Verification items for the finished model (mm, model axes). A direction names the side the tool comes from. Coordinates: 2 decimals unless noted, no trailing zeros. Loops run counter-clockwise (first coordinate to the right, second up) from the corner with the lowest first, then second, coordinate; pieces in that order, holes last.
Q1. Go/stop test with flat-tipped pins: P1, Ø8.5, axis at x = 5.5, y = 49, coming from the +Z side; P2, Ø4, axis at x = -18.85, y = -42.07, coming from the +Z side. Record where each tip stops, or that it passes through.
Q2. Material ranges on probe 1 along X at (y, z) = (94, 6.25); probe 2 along X at (y, z) = (140.5, 10.5); probe 3 along Y at (x, z) = (18, 12), recorded low to high.
Q3. Sectioned sample at A-A (z = 12.5). Count the separate pieces of the cut face and the enclosed holes in it, then the cut area to 3 significant figures.
Q4. Access from +Z, -Z, +X, -X, +Y, -Y to the whole of each face (thin tool, end or side, straight path). Record for faces 4 (the face through (17, 43, 7.938)), 5 (the face through (40.96, 65.94, 8.05)).
Q5. Mould release check, pull along Y, two halves, no side actions. Record for faces 1 (the face through (11, -52.388, 8)), 2 (the face through (10.282, 57.082, 4.024)), 3 (the face through (11, 143, 15.875)): +Y half, -Y half, draft (parallel to the pull), parting line (faces both ways), or undercut.
Q6. Sectioned sample at C-C (y = 54). Enter the section's corners in (x, z) (1 decimal), then the cut area to 3 significant figures.
Autodesk Inventor part; units mm, degrees
ref_plane "YZ Plane" through (0, 0, 0) normal (1, 0, 0) x (0, 1, 0)
ref_plane "XZ Plane" through (0, 0, 0) normal (0, 1, 0) x (-1, 0, 0)
ref_plane "XY Plane" through (0, 0, 0) normal (0, 0, 1) x (1, 0, 0)
sketch "Sketch1" plane through (0, 0, 0) normal (0, 0, 1) x (1, 0, 0)
  line L0 (-23.6094, 98.425) -> (-0.1834, 98.425)
  line L1 (-0.1834, 150.8125) -> (-0.1834, 98.425)
  line L2 (-23.6094, 150.8125) -> (-0.1834, 150.8125)
  line L3 (-23.6094, 150.8125) -> (-23.6094, 98.425)
  circle A0 centre (-18.8469, 140.4937) radius 2.3813
  circle A1 centre (-18.8469, 108.7437) radius 2.3812
  line L4 (-23.6094, -52.3875) -> (-0.1834, -52.3875)
  line L5 (-0.1834, 0) -> (-0.1834, -52.3875)
  line L6 (-23.6094, 0) -> (0, 0)
  line L7 (-23.6094, 0) -> (-23.6094, -52.3875)
  circle A2 centre (-18.8469, -10.3188) radius 2.3813
  circle A3 centre (-18.8469, -42.0688) radius 2.3813
  line L8 (22.8147, 98.425) -> (46.2406, 98.425)
  line L9 (46.2406, 150.8125) -> (46.2406, 98.425)
  line L10 (22.8147, 150.8125) -> (46.2406, 150.8125)
  line L11 (22.8147, 150.8125) -> (22.8147, 98.425)
  circle A4 centre (41.4781, 140.4938) radius 2.3813
  circle A5 centre (41.4781, 108.7438) radius 2.3813
  line L12 (22.8147, -52.3875) -> (46.2406, -52.3875)
  line L13 (46.2406, 0) -> (46.2406, -52.3875)
  line L14 (22.8147, 0) -> (46.2406, 0)
  line L15 (22.8147, 0) -> (22.8147, -52.3875)
  circle A6 centre (41.4781, -10.3187) radius 2.3813
  circle A7 centre (41.4781, -42.0687) radius 2.3813
  line L16 (22.8147, 150.8125) -> (-0.1834, 150.8125)
  line L17 (22.8147, -52.3875) -> (-0.1834, -52.3875)
  line L18 (46.2406, 0) -> (46.2406, 98.425)
  line L19 (-23.6094, 0) -> (-23.6094, 98.425)
extrude "Extrusion1" add sketch "Sketch1" along normal blind 15.875
sketch "Sketch2" plane through (-23.6094, -52.3875, 0) normal (-1, 0, 0) x (0, 0, 1)
  line L0 (15.875, 195.2625) -> (15.875, 190.5)
  line L1 (15.875, 163.5125) -> (15.875, 158.75)
  line L2 (15.875, 44.45) -> (15.875, 39.6875)
  line L3 (15.875, 190.5) -> (15.875, 163.5125) construction
  line L4 (15.875, 12.7) -> (0, 12.7) construction
  line L5 (15.875, 12.7) -> (15.875, 39.6875) construction
  line L6 (22.1465, 177.0062) -> (15.875, 177.0062)
  line L7 (15.875, 0) -> (15.875, 203.2)
  line L8 (24.8676, 26.1938) -> (15.875, 26.1938)
  line L9 (15.875, 203.2) -> (15.875, 0)
  circle A0 centre (15.875, 177.0062) radius 9.525
  circle A1 centre (15.875, 26.1938) radius 9.525
  point P0 (0, 52.3875)
  point P1 (15.875, 35.7188)
  point P2 (15.875, 16.6688)
  point P3 (15.875, 186.5312)
  point P4 (15.875, 167.4812)
  dimension "d2" = 19.05
  dimension "d3" = 19.05
extrude "Extrusion2" cut sketch "Sketch2" against normal blind 76.2 contours L7 A1 | A0 L7 picked at (15.1152, 19.9361) picked at (15.1152, 170.7485)
sketch "Sketch3" plane through (0, 0, 15.875) normal (0, 0, 1) x (1, 0, 0)
  circle A0 centre (41.4781, 108.7438) radius 2.3813 construction
  circle A1 centre (41.4781, -10.3187) radius 2.3813 construction
  line L0 (41.4781, 108.7438) -> (41.4781, -10.3187) construction
  circle A2 centre (41.4781, 49.2125) radius 2.3813 construction
  circle A3 centre (41.4781, 30.1625) radius 2.3813 construction
  circle A4 centre (41.4781, 68.2625) radius 2.3813 construction
  circle A5 centre (41.4781, 49.2125) radius 2.3813 construction
  circle A6 centre (41.4781, 68.2625) radius 2.3813
  circle A7 centre (41.4781, 49.2125) radius 2.3813
  circle A8 centre (41.4781, 30.1625) radius 2.3813
  point P0 (0, 0)
  dimension "d8" = 19.05
  dimension "d11" = 19.05
extrude "Extrusion3" cut sketch "Sketch3" against normal blind 76.2
sketch "Sketch4" plane through (0, 0, 15.875) normal (0, 0, 1) x (1, 0, 0)
  circle A0 centre (11.3156, 49.2125) radius 14.2875
  line L0 (-23.6094, 115.0937) -> (-23.6094, -16.6688)
  point P0 (0, 0)
  dimension "d16" = 34.925
  dimension "d17" = 28.575
extrude "Extrusion4" cut sketch "Sketch4" against normal blind 7.9375
sketch "Sketch5" plane through (11.3156, 49.2125, 7.9375) normal (0, 0, 1) x (1, 0, 0)
  circle A0 centre (0, 0) radius 7.9375
  point P0 (-11.3156, -49.2125)
  dimension "d20" = 15.875
extrude "Extrusion5" cut sketch "Sketch5" against normal blind 7.9375
sketch "Sketch6" plane through (0, 0, 15.875) normal (0, 0, 1) x (1, 0, 0)
  line L0 (-23.6094, 100.0125) -> (46.2406, 100.0125)
  line L1 (46.2406, -1.5875) -> (-23.6094, -1.5875)
  circle A0 centre (11.3156, 49.2125) radius 37.465
  circle A1 centre (40.3188, 93.6625) radius 2.3813
  line L2 (48.7806, 49.2125) -> (-26.1494, 49.2125) construction
  line L3 (11.3156, 100.0125) -> (11.3156, -1.5875) construction
  circle A2 centre (40.3188, 4.7625) radius 2.3813
  circle A3 centre (-17.6876, 93.6625) radius 2.3813
  circle A4 centre (-17.6876, 4.7625) radius 2.3813
  point P0 (0, 0)
  dimension "d23" = 4.7625
  dimension "d24" = 6.35
extrude "Extrusion6" cut sketch "Sketch6" against normal blind 19.05 contours A1 | A2 | A3 | A4
sketch "Sketch7" plane through (0, 0, 0) normal (0, 0, -1) x (-1, 0, 0)
  point P0 (0, 0)
properties part number "YClamp"
Geometry check:
1. P1: stops at z = 7.94
1. P2: passes through
2. probe 1: x = -23.61 to -20.04, -15.33 to 37.96, 42.68 to 46.24
2. probe 2: x = -23.61 to -21.23, -16.47 to 39.1, 43.86 to 46.24
2. probe 3: y = -52.39 to -34.89, -17.49 to 36.59, 61.84 to 115.92, 133.32 to 150.81
3. separate pieces: 3
3. enclosed holes: 16
3. area: 10,800 mm2
4. face 4: +Z
4. face 5: +Z, -Z
5. face 1: -Y half
5. face 2: undercut
5. face 3: draft
6. outline: (-23.6, 0) - (5, 0) - (5, 7.9) - (-2.1, 7.9) - (-2.1, 15.9) - (-23.6, 15.9) - close; (17.6, 0) - (46.2, 0) - (46.2, 15.9) - (24.8, 15.9) - (24.8, 7.9) - (17.6, 7.9) - close
6. area: 795 mm2
